Part model, mm, in its own coordinate system. Round coordinates to 2 decimals unless told otherwise and drop trailing zeros. Loops run counter-clockwise (first coordinate to the right, second up) from the corner with the lowest first, then second, coordinate; pieces in that order, holes last. Notation, with made-up numbers: M -19,-26 L 36,-26 A19 cw 36,-2 Z; hole C 50,-25 d2. An arc over 180 degrees is marked long. Put each result on its own line as item: value. Start each with the question number.
1) Slice it at A-A on z = -54. Give the cut face in (x, y), then the cut area to 3 significant figures.
2) Probe line 1 along X through (y, z) = (2.25, -2); line 2 along Z through (x, y) = (-48, 3); line 3 along Z through (x, y) = (-0.5, 0.75). List the from-to ranges inside material, lowest first.
3) Slice it at C-C on x = 0. State how many separate pieces and enclosed holes the cut face has, then the cut area to 3 significant figures.
4) Drop flat-ended pins along their axis: pin 1 Ø2 at (y, z) = (1.5, -35) entering from +X; pin 2 Ø4 at (x, y) = (-40, 4) entering from +Z; pin 3 Ø3 at (x, z) = (-17.22, -41.57) entering from +Y; pin 4 Ø3 at (y, z) = (3, -24.5) entering from -X. Give the stop position or say it passes through.
5) Slice it at B-B on x = 54. Give the cut face in (y, z).
```python
from build123d import *

# Parameters (mm, degrees)
SKETCH1_R           = 57.5
SKETCH1_R_2         = 1.75
SKETCH1_R_3         = 26
SKETCH1_R_4         = 2.5
BOSS_EXTRUDE1_DEPTH = 7
SKETCH2_R           = 7
SKETCH2_R_2         = 5
CUT_EXTRUDE1_DEPTH  = 1


with BuildPart() as part:
    # Sketch1 → Boss-Extrude1 (new body)
    with BuildSketch(Plane(origin=(0, 0, 0), x_dir=(1, 0, 0), z_dir=(0, 1, 0))):
        with Locations(Location((0, 0, 0), (0, 0, 270))):
            Circle(SKETCH1_R)
        with Locations(Location((0, 54, 0), (0, 0, 270))):
            Circle(SKETCH1_R_2, mode=Mode.SUBTRACT)
        with Locations(Location((27, 46.765371804, 0), (0, 0, 270))):
            Circle(SKETCH1_R_2, mode=Mode.SUBTRACT)
        with Locations(Location((46.765371804, 27, 0), (0, 0, 270))):
            Circle(SKETCH1_R_2, mode=Mode.SUBTRACT)
        with Locations(Location((54, 0, 0), (0, 0, 270))):
            Circle(SKETCH1_R_2, mode=Mode.SUBTRACT)
        with Locations(Location((46.765371804, -27, 0), (0, 0, 270))):
            Circle(SKETCH1_R_2, mode=Mode.SUBTRACT)
        with Locations(Location((27, -46.765371804, 0), (0, 0, 270))):
            Circle(SKETCH1_R_2, mode=Mode.SUBTRACT)
        with Locations(Location((0, -54, 0), (0, 0, 270))):
            Circle(SKETCH1_R_2, mode=Mode.SUBTRACT)
        with Locations(Location((-27, -46.765371804, 0), (0, 0, 270))):
            Circle(SKETCH1_R_2, mode=Mode.SUBTRACT)
        with Locations(Location((-46.765371804, -27, 0), (0, 0, 270))):
            Circle(SKETCH1_R_2, mode=Mode.SUBTRACT)
        with Locations(Location((-54, 0, 0), (0, 0, 270))):
            Circle(SKETCH1_R_2, mode=Mode.SUBTRACT)
        with Locations(Location((-46.765371804, 27, 0), (0, 0, 270))):
            Circle(SKETCH1_R_2, mode=Mode.SUBTRACT)
        with Locations(Location((-27, 46.765371804, 0), (0, 0, 270))):
            Circle(SKETCH1_R_2, mode=Mode.SUBTRACT)
        with Locations(Location((0, 0, 0), (0, 0, 270))):
            Circle(SKETCH1_R_3, mode=Mode.SUBTRACT)
        with Locations(Location((0, 45, 0), (0, 0, 270))):
            Circle(SKETCH1_R_4, mode=Mode.SUBTRACT)
        with Locations(Location((17.220754456, 41.574578963, 0), (0, 0, 270))):
            Circle(SKETCH1_R_4, mode=Mode.SUBTRACT)
        with Locations(Location((31.819805153, 31.819805153, 0), (0, 0, 270))):
            Circle(SKETCH1_R_4, mode=Mode.SUBTRACT)
        with Locations(Location((41.574578963, 17.220754456, 0), (0, 0, 270))):
            Circle(SKETCH1_R_4, mode=Mode.SUBTRACT)
        with Locations(Location((45, 0, 0), (0, 0, 270))):
            Circle(SKETCH1_R_4, mode=Mode.SUBTRACT)
        with Locations(Location((41.574578963, -17.220754456, 0), (0, 0, 270))):
            Circle(SKETCH1_R_4, mode=Mode.SUBTRACT)
        with Locations(Location((31.819805153, -31.819805153, 0), (0, 0, 270))):
            Circle(SKETCH1_R_4, mode=Mode.SUBTRACT)
        with Locations(Location((17.220754456, -41.574578963, 0), (0, 0, 270))):
            Circle(SKETCH1_R_4, mode=Mode.SUBTRACT)
        with Locations(Location((0, -45, 0), (0, 0, 270))):
            Circle(SKETCH1_R_4, mode=Mode.SUBTRACT)
        with Locations(Location((-17.220754456, -41.574578963, 0), (0, 0, 270))):
            Circle(SKETCH1_R_4, mode=Mode.SUBTRACT)
        with Locations(Location((-31.819805153, -31.819805153, 0), (0, 0, 270))):
            Circle(SKETCH1_R_4, mode=Mode.SUBTRACT)
        with Locations(Location((-41.574578963, -17.220754456, 0), (0, 0, 270))):
            Circle(SKETCH1_R_4, mode=Mode.SUBTRACT)
        with Locations(Location((-45, 0, 0), (0, 0, 270))):
            Circle(SKETCH1_R_4, mode=Mode.SUBTRACT)
        with Locations(Location((-41.574578963, 17.220754456, 0), (0, 0, 270))):
            Circle(SKETCH1_R_4, mode=Mode.SUBTRACT)
        with Locations(Location((-31.819805153, 31.819805153, 0), (0, 0, 270))):
            Circle(SKETCH1_R_4, mode=Mode.SUBTRACT)
        with Locations(Location((-17.220754456, 41.574578963, 0), (0, 0, 270))):
            Circle(SKETCH1_R_4, mode=Mode.SUBTRACT)
    extrude(amount=BOSS_EXTRUDE1_DEPTH)

    # Sketch2 → Cut-Extrude1 (cut)
    # profile 1 of 16: a face of its own
    with BuildSketch(Plane(origin=(0, 7, 0), x_dir=(1, 0, 0), z_dir=(0, 1, 0))):
        with Locations(Location((0, 45, 0), (0, 0, 270))):
            Circle(SKETCH2_R)
        with Locations(Location((0, 45, 0), (0, 0, 270))):
            Circle(SKETCH2_R_2, mode=Mode.SUBTRACT)
    # profile 2 of 16: a face of its own
    with BuildSketch(Plane(origin=(0, 7, 0), x_dir=(1, 0, 0), z_dir=(0, 1, 0))):
        with Locations(Location((17.220754456, 41.574578963, 0), (0, 0, 270))):
            Circle(SKETCH2_R)
        with Locations(Location((17.220754456, 41.574578963, 0), (0, 0, 270))):
            Circle(SKETCH2_R_2, mode=Mode.SUBTRACT)
    # profile 3 of 16: a face of its own
    with BuildSketch(Plane(origin=(0, 7, 0), x_dir=(1, 0, 0), z_dir=(0, 1, 0))):
        with Locations(Location((31.819805153, 31.819805153, 0), (0, 0, 270))):
            Circle(SKETCH2_R)
        with Locations(Location((31.819805153, 31.819805153, 0), (0, 0, 270))):
            Circle(SKETCH2_R_2, mode=Mode.SUBTRACT)
    # profile 4 of 16: a face of its own
    with BuildSketch(Plane(origin=(0, 7, 0), x_dir=(1, 0, 0), z_dir=(0, 1, 0))):
        with Locations(Location((41.574578963, 17.220754456, 0), (0, 0, 270))):
            Circle(SKETCH2_R)
        with Locations(Location((41.574578963, 17.220754456, 0), (0, 0, 270))):
            Circle(SKETCH2_R_2, mode=Mode.SUBTRACT)
    # profile 5 of 16: a face of its own
    with BuildSketch(Plane(origin=(0, 7, 0), x_dir=(1, 0, 0), z_dir=(0, 1, 0))):
        with Locations(Location((45, 0, 0), (0, 0, 270))):
            Circle(SKETCH2_R)
        with Locations(Location((45, 0, 0), (0, 0, 270))):
            Circle(SKETCH2_R_2, mode=Mode.SUBTRACT)
    # profile 6 of 16: a face of its own
    with BuildSketch(Plane(origin=(0, 7, 0), x_dir=(1, 0, 0), z_dir=(0, 1, 0))):
        with Locations(Location((41.574578963, -17.220754456, 0), (0, 0, 270))):
            Circle(SKETCH2_R)
        with Locations(Location((41.574578963, -17.220754456, 0), (0, 0, 270))):
            Circle(SKETCH2_R_2, mode=Mode.SUBTRACT)
    # profile 7 of 16: a face of its own
    with BuildSketch(Plane(origin=(0, 7, 0), x_dir=(1, 0, 0), z_dir=(0, 1, 0))):
        with Locations(Location((31.819805153, -31.819805153, 0), (0, 0, 270))):
            Circle(SKETCH2_R)
        with Locations(Location((31.819805153, -31.819805153, 0), (0, 0, 270))):
            Circle(SKETCH2_R_2, mode=Mode.SUBTRACT)
    # profile 8 of 16: a face of its own
    with BuildSketch(Plane(origin=(0, 7, 0), x_dir=(1, 0, 0), z_dir=(0, 1, 0))):
        with Locations(Location((17.220754456, -41.574578963, 0), (0, 0, 270))):
            Circle(SKETCH2_R)
        with Locations(Location((17.220754456, -41.574578963, 0), (0, 0, 270))):
            Circle(SKETCH2_R_2, mode=Mode.SUBTRACT)
    # profile 9 of 16: a face of its own
    with BuildSketch(Plane(origin=(0, 7, 0), x_dir=(1, 0, 0), z_dir=(0, 1, 0))):
        with Locations(Location((0, -45, 0), (0, 0, 270))):
            Circle(SKETCH2_R)
        with Locations(Location((0, -45, 0), (0, 0, 270))):
            Circle(SKETCH2_R_2, mode=Mode.SUBTRACT)
    # profile 10 of 16: a face of its own
    with BuildSketch(Plane(origin=(0, 7, 0), x_dir=(1, 0, 0), z_dir=(0, 1, 0))):
        with Locations(Location((-17.220754456, -41.574578963, 0), (0, 0, 270))):
            Circle(SKETCH2_R)
        with Locations(Location((-17.220754456, -41.574578963, 0), (0, 0, 270))):
            Circle(SKETCH2_R_2, mode=Mode.SUBTRACT)
    # profile 11 of 16: a face of its own
    with BuildSketch(Plane(origin=(0, 7, 0), x_dir=(1, 0, 0), z_dir=(0, 1, 0))):
        with Locations(Location((-31.819805153, -31.819805153, 0), (0, 0, 270))):
            Circle(SKETCH2_R)
        with Locations(Location((-31.819805153, -31.819805153, 0), (0, 0, 270))):
            Circle(SKETCH2_R_2, mode=Mode.SUBTRACT)
    # profile 12 of 16: a face of its own
    with BuildSketch(Plane(origin=(0, 7, 0), x_dir=(1, 0, 0), z_dir=(0, 1, 0))):
        with Locations(Location((-41.574578963, -17.220754456, 0), (0, 0, 270))):
            Circle(SKETCH2_R)
        with Locations(Location((-41.574578963, -17.220754456, 0), (0, 0, 270))):
            Circle(SKETCH2_R_2, mode=Mode.SUBTRACT)
    # profile 13 of 16: a face of its own
    with BuildSketch(Plane(origin=(0, 7, 0), x_dir=(1, 0, 0), z_dir=(0, 1, 0))):
        with Locations(Location((-45, 0, 0), (0, 0, 270))):
            Circle(SKETCH2_R)
        with Locations(Location((-45, 0, 0), (0, 0, 270))):
            Circle(SKETCH2_R_2, mode=Mode.SUBTRACT)
    # profile 14 of 16: a face of its own
    with BuildSketch(Plane(origin=(0, 7, 0), x_dir=(1, 0, 0), z_dir=(0, 1, 0))):
        with Locations(Location((-41.574578963, 17.220754456, 0), (0, 0, 270))):
            Circle(SKETCH2_R)
        with Locations(Location((-41.574578963, 17.220754456, 0), (0, 0, 270))):
            Circle(SKETCH2_R_2, mode=Mode.SUBTRACT)
    # profile 15 of 16: a face of its own
    with BuildSketch(Plane(origin=(0, 7, 0), x_dir=(1, 0, 0), z_dir=(0, 1, 0))):
        with Locations(Location((-31.819805153, 31.819805153, 0), (0, 0, 270))):
            Circle(SKETCH2_R)
        with Locations(Location((-31.819805153, 31.819805153, 0), (0, 0, 270))):
            Circle(SKETCH2_R_2, mode=Mode.SUBTRACT)
    # profile 16 of 16: a face of its own
    with BuildSketch(Plane(origin=(0, 7, 0), x_dir=(1, 0, 0), z_dir=(0, 1, 0))):
        with Locations(Location((-17.220754456, 41.574578963, 0), (0, 0, 270))):
            Circle(SKETCH2_R)
        with Locations(Location((-17.220754456, 41.574578963, 0), (0, 0, 270))):
            Circle(SKETCH2_R_2, mode=Mode.SUBTRACT)
    extrude(amount=-CUT_EXTRUDE1_DEPTH, mode=Mode.SUBTRACT)


solid = part.part
```
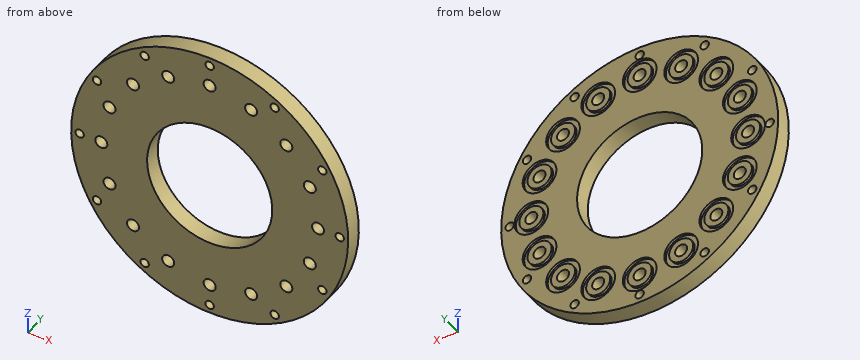
Recorded:
1. outline: M -19.75,0 L -1.75,0 L -1.75,7 L -19.75,7 Z; M 1.75,0 L 19.75,0 L 19.75,7 L 1.75,7 Z
1. area: 252 mm2
2. line 1: x = -57.47 to -46.5, -43.5 to -25.92, 25.92 to 43.5, 46.5 to 57.47
2. line 2: z = -31.66 to -28.24, -25.76 to 25.76, 28.24 to 31.66
2. line 3: z = -57.5 to -55.68, -52.32 to -47.45, -42.55 to -26, 26 to 42.55, 47.45 to 52.32, 55.68 to 57.5
3. separate pieces: 6
3. enclosed holes: 0
3. area: 314 mm2
4. pin 1: stops at x = 46.37
4. pin 2: stops at z = 43.15
4. pin 3: passes through
4. pin 4: stops at x = -52.7
5. outline: M 0,-19.75 L 7,-19.75 L 7,-1.75 L 0,-1.75 Z; M 0,1.75 L 7,1.75 L 7,19.75 L 0,19.75 Z
